Part print with two shaded views. Sizes in mm from the minimum x, y, z corner. A direction names the side the tool comes from. Coordinates: 2 decimals unless noted, no trailing zeros. Loops run counter-clockwise (first coordinate to the right, second up) from the corner with the lowest first, then second, coordinate; pieces in that order, holes last.
Item 1: 3-axis set-ups, long thin cutter, end or side, ignore diameter. For the marked faces 1, 2 and 3: which of +Z, -Z, +X, -X, +Y, -Y reach the whole face in a straight line?
Item 2: Drill centre lines: line 1 along X through (y, z) = (26, 1.75); line 2 along X through (y, z) = (59, 4.45); line 3 along X through (y, z) = (9, 3.9). Where is each one in solid material? Low to high.
Item 3: Cut at C-C (z = 4). Count the separate pieces of the cut face and the enclosed holes in it, and give its area (3 significant figures).
Item 4: Mould opens along X. For the marked faces 4, 5, 6 and 7 say: released by +X, released by -X, zero draft, split by the parting line, or undercut.
Item 5: Flat gauge pins, fed straight in: pin 1 (1.5 mm diameter, centred on x = 27, z = 3, fed in from -Y); pin 2 (1.5 mm diameter, centred on x = 14.5, z = 3, fed in from -Y); pin 3 (2.5 mm diameter, centred on y = 66.5, z = 1.5, fed in from -X); pin 4 (2 mm diameter, centred on x = 20.5, z = 4, fed in from -Y). Where does each tip first touch, or does it go through?
Item 6: Cut at B-B (y = 21). List the corners of the cut face in (x, z).
Item 7: Cut at D-D (x = 11.75). List the corners of the cut face in (y, z), and give its area (3 significant figures).
Item 8: Cut at A-A (y = 12). List the corners of the cut face in (x, z), and give its area (3 significant figures).
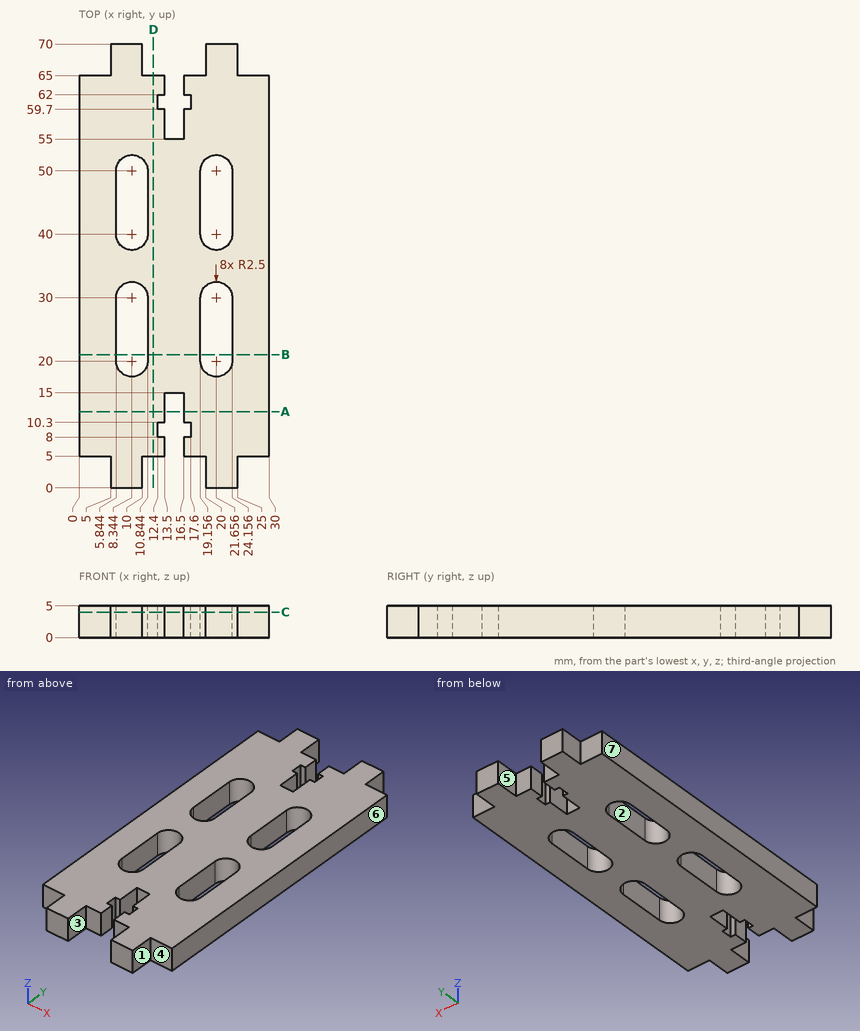
Filled sheet:
1. face 1: +Z, -Z, +X, -Y
1. face 2: +Z, -Z
1. face 3: +Z, -Z, -Y
2. line 1: x = 0 to 5.84, 10.84 to 19.16, 24.16 to 30
2. line 2: x = 0 to 13.5, 16.5 to 30
2. line 3: x = 0 to 12.4, 17.6 to 30
3. separate pieces: 1
3. enclosed holes: 4
3. area: 1,550 mm2
4. face 4: zero draft
4. face 5: undercut
4. face 6: released by +X
4. face 7: released by -X
5. pin 1: stops at y = 5
5. pin 2: stops at y = 15
5. pin 3: stops at x = 5
5. pin 4: stops at y = 0
6. outline: (0, 0) - (5.84, 0) - (5.84, 5) - (0, 5) - close; (10.84, 0) - (19.16, 0) - (19.16, 5) - (10.84, 5) - close; (24.16, 0) - (30, 0) - (30, 5) - (24.16, 5) - close
7. outline: (5, 0) - (65, 0) - (65, 5) - (5, 5) - close
7. area: 300 mm2
8. outline: (0, 0) - (13.5, 0) - (13.5, 5) - (0, 5) - close; (16.5, 0) - (30, 0) - (30, 5) - (16.5, 5) - close
8. area: 135 mm2
